```python
from build123d import *

# Parameters (mm, degrees)
ESQUISSE1_W        = 50
ESQUISSE1_H        = 55
BOSS_EXTRU_1_DEPTH = 37
ESQUISSE2_R        = 7.5
BOSS_EXTRU_2_DEPTH = 10
CONG_3_R           = 2


with BuildPart() as part:
    # Esquisse1 → Boss.-Extru.1 (new body)
    with BuildSketch(Plane.XY):
        Rectangle(ESQUISSE1_W, ESQUISSE1_H)
    extrude(amount=BOSS_EXTRU_1_DEPTH)

    # Esquisse2 → Boss.-Extru.2 (add)
    with BuildSketch(Plane.XY):
        Circle(ESQUISSE2_R)
    extrude(amount=-BOSS_EXTRU_2_DEPTH)

    # Congé3
    cong_3_edges = [part.edges().sort_by_distance(p)[0] for p in [
        (-7.5, 0, -10),
    ]]
    fillet(cong_3_edges, radius=CONG_3_R)


solid = part.part
```
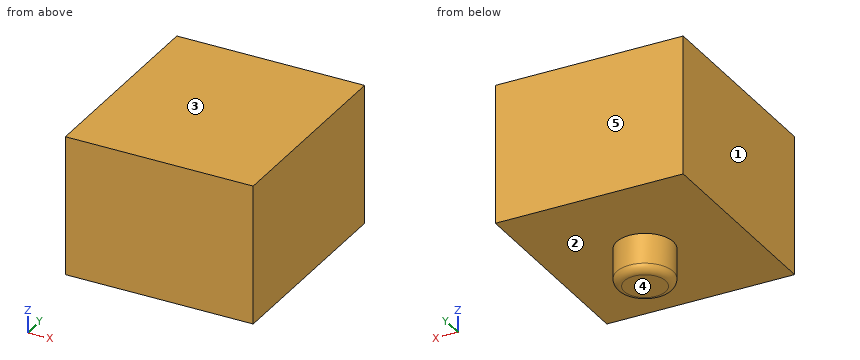
Model file for the job. Use its own axes, mm. Face numbers are marked on the shaded views. A direction names the side the tool comes from. Give positions to 0.01 mm unless a question says otherwise; leave off trailing zeros. Write each loop counter-clockwise with the first axis right and the second up, starting at its lowest first coordinate (ties: lowest second). Pieces come first, ordered by that corner, then holes. Notation, with made-up numbers: M -26.5,43.5 L 28.5,43.5 A25 ccw 28.5,62.5 Z; hole C 26.25,-15.5 d10. An arc over 180 degrees is marked long. Use a Markdown table: item, result.
1) Drill centre lines: line 1 (Z direction, x = -11, y = -24.5); line 2 (Z direction, x = -1, y = 6). Where is each one in solid material? Low to high. Write a range as from..to.
Responses:
| item | result |
|---|---|
| line 1 | z = 0..37 |
| line 2 | z = -9.91..37 |
2) Cut at C-C (z = -3.5). List the corners of the cut face in (x, y).
Responses:
| item | result |
|---|---|
| outline | C 0,0 d15 |
3) Tool access for the marked faces 1 and 2: list every direction of +Z, -Z, +X, -X, +Y, -Y with a clear straight run to the whole face (end or side of a thin tool).
Responses:
| item | result |
|---|---|
| face 1 | +Z, -Z, -X, +Y, -Y |
| face 2 | -Z |
4) Cut at D-D (y = 15). List the corners of the cut face in (x, z), and give its area (3 significant figures).
Responses:
| item | result |
|---|---|
| outline | M -25,0 L 25,0 L 25,37 L -25,37 Z |
| area | 1,850 mm2 |
5) Cut at A-A (y = 0). List the corners of the cut face in (x, z), and give its area (3 significant figures).
Responses:
| item | result |
|---|---|
| outline | M -25,0 L -7.5,0 L -7.5,-8 A2 ccw -5.5,-10 L 5.5,-10 A2 ccw 7.5,-8 L 7.5,0 L 25,0 L 25,37 L -25,37 Z |
| area | 2,000 mm2 |
6) Pull direction Z, two halves, no side cores. Call the marked faces 3, 4 and 5: +Z half, -Z half, draft (parallel to the pull), parting line (faces both ways), or undercut.
Responses:
| item | result |
|---|---|
| face 3 | +Z half |
| face 4 | -Z half |
| face 5 | draft |
7) Cut at B-B (x = 0). List the corners of the cut face in (y, z), and give its area (3 significant figures).
Responses:
| item | result |
|---|---|
| outline | M -27.5,0 L -7.5,0 L -7.5,-8 A2 ccw -5.5,-10 L 5.5,-10 A2 ccw 7.5,-8 L 7.5,0 L 27.5,0 L 27.5,37 L -27.5,37 Z |
| area | 2,180 mm2 |
